Verification items for the finished model (mm, model axes). Face numbers are marked on the shaded views. Round coordinates to 2 decimals unless told otherwise and drop trailing zeros. Loops run counter-clockwise (first coordinate to the right, second up) from the corner with the lowest first, then second, coordinate; pieces in that order, holes last. Notation, with made-up numbers: M 49.5,31.5 L 54.5,31.5 A22 cw 54.5,41.5 Z; hole C 71,-12.5 d5. An arc over 180 degrees is marked long. One line per item, written item: value.
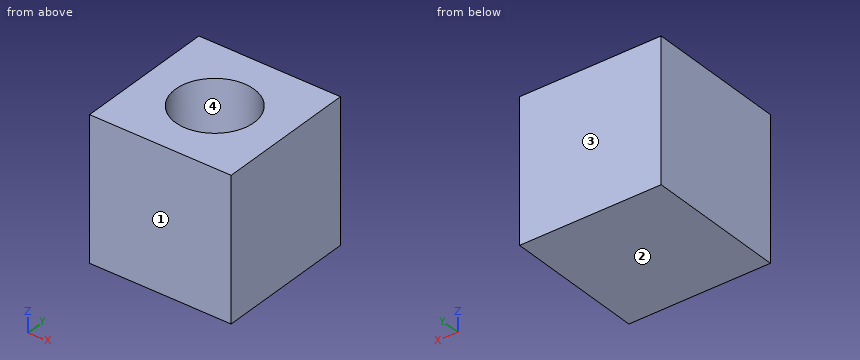
from build123d import *

# Parameters (mm, degrees)
F1_W     = 50
F1_H     = 50
F2_DEPTH = 50
F4_D     = 27.7
F4_DEPTH = 30
F4_TIP   = 8.3219195735


with BuildPart() as f2:
    # F1 (on face) → F2 (new body)
    with BuildSketch(Plane.XZ):
        with Locations((25, 25)):
            Rectangle(F1_W, F1_H)
    extrude(amount=F2_DEPTH)

    # F4
    with Locations(Plane.XY.offset(50)):
        with Locations((25, -25.1106228679)):
            Hole(F4_D / 2, depth=F4_DEPTH)
            with Locations((0, 0, -(F4_DEPTH + F4_TIP / 2))):  # 118° drill point
                Cone(0, F4_D / 2, F4_TIP, mode=Mode.SUBTRACT)


solid = f2.part
(1) Sectioned sample at A-A on z = 25. Enter the section's corners in (x, y), and give its area (3 significant figures).
Completed:
outline: M 0,-50 L 50,-50 L 50,0 L 0,0 Z; hole C 25,-25.11 d27.7
area: 1,900 mm^2
(2) Thickness scan on L1, parallel to Y at x = 25, z = 43.5; L2, parallel to Y at x = 35.5, z = 21; L3, parallel to X at y = -29, z = 33. Record the ranges inside material, lowest first. Write a range as from..to.
Completed:
L1: y = -50..-38.96, -11.26..0
L2: y = -50..-34.14, -16.08..0
L3: x = 0..11.71, 38.29..50
(3) Sectioned sample at B-B on z = 14. Enter the section's corners in (x, y), and give its area (3 significant figures).
Completed:
outline: M 0,-50 L 50,-50 L 50,0 L 0,0 Z; hole C 25,-25.11 d7.73
area: 2,450 mm^2
(4) Mould release check, pull along Y, two halves, no side actions. Record for the marked faces 1, 2, 3 and 4: +Y half, -Y half, draft (parallel to the pull), parting line (faces both ways), or undercut.
Completed:
face 1: -Y half
face 2: draft
face 3: +Y half
face 4: undercut
